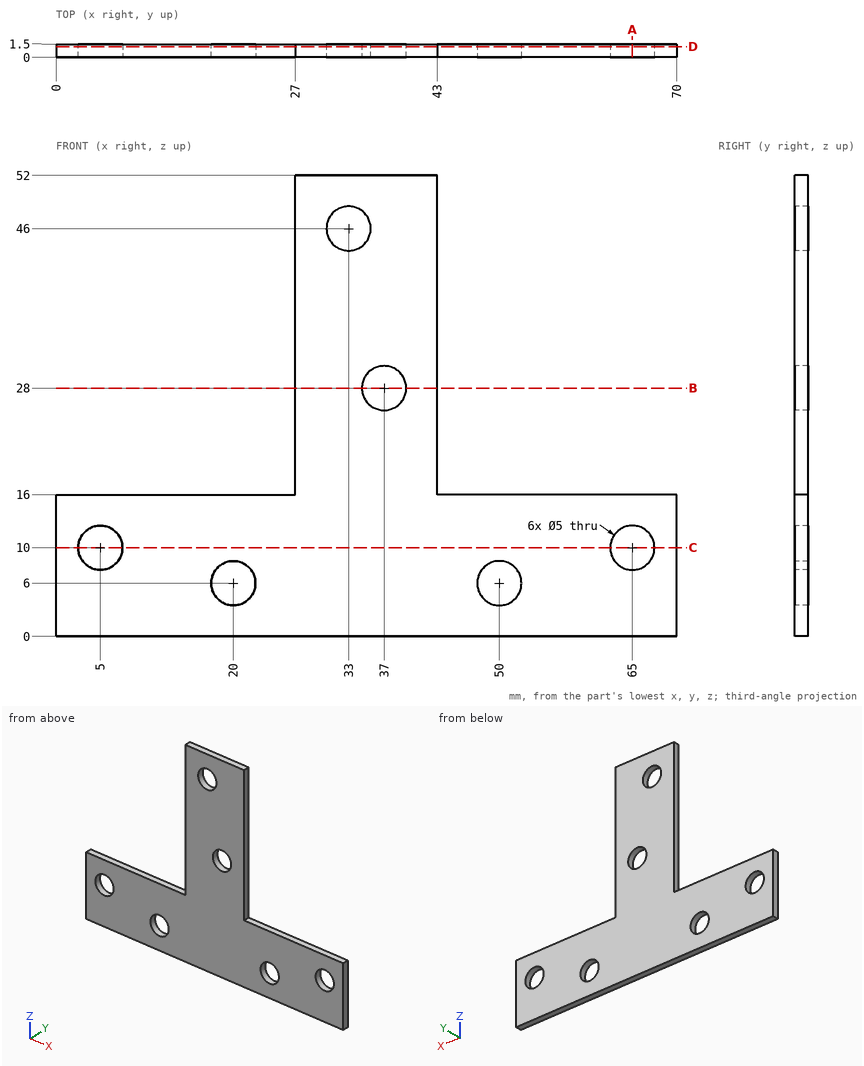
Input: dimensioned drawing with shaded views. Units: mm. Origin: part minimum x, y, z. Coordinates: 2 decimals unless noted, no trailing zeros. Write each loop counter-clockwise with the first axis right and the second up, starting at its lowest first coordinate (ties: lowest second). Pieces come first, ordered by that corner, then holes. Notation, with made-up numbers: M 57,28 L 111,28 A20 cw 111,53 Z; hole C 53,-27.75 d3. An arc over 180 degrees is marked long. Answer as CSV lines item,"result". Start each with the question number.
Q1. Cut plane D-D on y = 1.2. Return the cut outline in (x, z), then the cut area to 3 significant figures.
Q2. Pin query (flat end, axial travel): P1, Ø0.8, axis at y = 0.5, z = 35, coming from the +X side. Return the tip coordinate at first contact, or that it passes through.
Q3. Cut plane A-A on x = 65. Return the cut outline in (y, z), then the cut area to 3 significant figures.
Q4. Cut plane C-C on z = 10. Return the cut outline in (x, y), then the cut area to 3 significant figures.
Q5. Cut plane B-B on z = 28. Return the cut outline in (x, y), then the cut area to 3 significant figures.
Q6. Line query: line 1 (Z direction, x = 20, y = 0.85); line 2 (Z direction, x = 5, y = 1.25); line 3 (Z direction, x = 35, y = 0.3). Output: solid intervals per line, ascending. Write a range as from..to.
Findings below:
1,outline,"M 0,0 L 70,0 L 70,16 L 43,16 L 43,52 L 27,52 L 27,16 L 0,16 Z; hole C 5,10 d5; hole C 20,6 d5; hole C 33,46 d5; hole C 37,28 d5; hole C 50,6 d5; hole C 65,10 d5"
1,area,"1,580 mm2"
2,P1,"stops at x = 43"
3,outline,"M 0,0 L 1.5,0 L 1.5,7.5 L 0,7.5 Z; M 0,12.5 L 1.5,12.5 L 1.5,16 L 0,16 Z"
3,area,"16.5 mm2"
4,outline,"M 0,0 L 2.5,0 L 2.5,1.5 L 0,1.5 Z; M 7.5,0 L 62.5,0 L 62.5,1.5 L 7.5,1.5 Z; M 67.5,0 L 70,0 L 70,1.5 L 67.5,1.5 Z"
4,area,"90.0 mm2"
5,outline,"M 27,0 L 34.5,0 L 34.5,1.5 L 27,1.5 Z; M 39.5,0 L 43,0 L 43,1.5 L 39.5,1.5 Z"
5,area,"16.5 mm2"
6,line 1,"z = 0..3.5, 8.5..16"
6,line 2,"z = 0..7.5, 12.5..16"
6,line 3,"z = 0..26.5, 29.5..44.5, 47.5..52"
